Geometry check sheet. Reference: the model listing, model coordinates, mm. Face numbers are marked on the shaded views. A direction names the side the tool comes from. Round coordinates to 2 decimals unless told otherwise and drop trailing zeros. Order: outer loops, then holes, each group sorted by start corner. A loop starts at its lowest first (then second) coordinate and runs counter-clockwise, first axis right, second up. Notation, with made-up numbers: (28, 7) - (53, 7) arc R12 cw to (53, 19) - close; hole circle Ø11 at (59.25, 44). An arc over 180 degrees is marked (long way). Return JSON: item names as keys, results as strings. Group by question number.
Q1. Sectioned sample at B-B, the plane y = 42. Record the cut outline in (x, z).
Q2. Sectioned sample at C-C, the plane z = 4. Record the cut outline in (x, y).
Q3. Sectioned sample at D-D, the plane x = -6.5. Record the cut outline in (y, z).
Q4. Material ranges on line 1 along Y through (x, z) = (-4.25, -5); line 2 along Z through (x, y) = (-6.25, 16.5); line 3 along X through (y, z) = (48, 1.75), recorded low to high.
Q5. Gauge pin test, flat ends, axial feed: pin 1 Ø4 at (y, z) = (21.5, 4) entering from -X; pin 2 Ø3 at (y, z) = (28.5, 2.5) entering from +X (3 decimals); pin 3 Ø2 at (y, z) = (28.5, -3) entering from +X. Record the tip position at first contact, or that the pin passes through.
Q6. Tool access check on the marked faces 1, 2 and 3. Record the directions out of +Z, -Z, +X, -X, +Y, -Y that give a thin tool (end or side, any length) a straight path to the whole face; none if there is none.
Q7. Sectioned sample at A-A, the plane x = 0. Record the cut outline in (y, z), then the cut area to 3 significant figures.
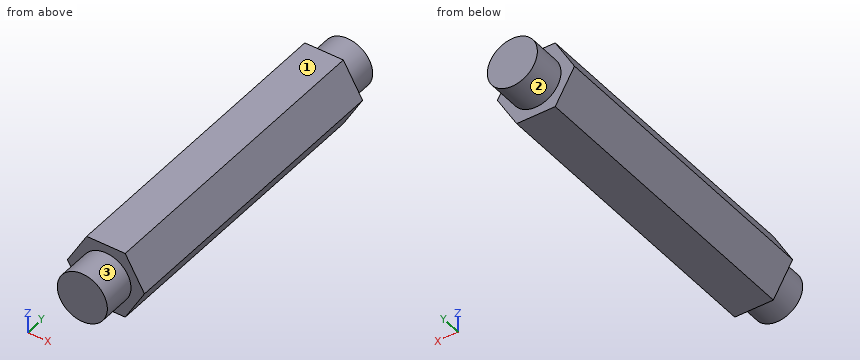
```python
from build123d import *

# Parameters (mm, degrees)
SALIENTE_EXTRUIR1_DEPTH = 58.68
CROQUIS2_R              = 4.7625
SALIENTE_EXTRUIR2_DEPTH = 6.35
SALIENTE_EXTRUIR3_START = 6.35
CROQUIS3_R              = 4.7625
SALIENTE_EXTRUIR3_DEPTH = 6.35


with BuildPart() as part:
    # Croquis1 → Saliente-Extruir1 (new body)
    with BuildSketch(Plane(origin=(0, 0, 0), x_dir=(1, 0, 0), z_dir=(0, 1, 0))):
        Polygon((7.332348419, 0), (3.666174209, 6.35), (-3.666174209, 6.35), (-7.332348419, 0), (-3.666174209, -6.35), (3.666174209, -6.35), align=None)
    extrude(amount=SALIENTE_EXTRUIR1_DEPTH)

    # Croquis2 → Saliente-Extruir2 (add)
    with BuildSketch(Plane(origin=(0, 58.68, 0), x_dir=(1, 0, 0), z_dir=(0, 1, 0))):
        with Locations(Location((0, 0, 0), (0, 0, 270))):
            Circle(CROQUIS2_R)
    extrude(amount=SALIENTE_EXTRUIR2_DEPTH)

    # Croquis3 → Saliente-Extruir3 (add)
    with BuildSketch(Plane.XZ.offset(SALIENTE_EXTRUIR3_START)):
        with Locations(Location((0, 0, 0), (0, 0, 90))):
            Circle(CROQUIS3_R)
    extrude(amount=-SALIENTE_EXTRUIR3_DEPTH)


solid = part.part
```
Reply:
{
 "1": {"outline": "(-7.33, 0) - (-3.67, -6.35) - (3.67, -6.35) - (7.33, 0) - (3.67, 6.35) - (-3.67, 6.35) - close"},
 "2": {"outline": "(-5.02, 0) - (-2.58, 0) - (-2.58, -6.35) - (2.58, -6.35) - (2.58, 0) - (5.02, 0) - (5.02, 58.68) - (2.58, 58.68) - (2.58, 65.03) - (-2.58, 65.03) - (-2.58, 58.68) - (-5.02, 58.68) - close"},
 "3": {"outline": "(0, -1.44) - (58.68, -1.44) - (58.68, 1.44) - (0, 1.44) - close"},
 "4": {"line 1": "0 to 58.68", "line 2": "-1.87 to 1.87", "line 3": "-6.32 to 6.32"},
 "5": {"pin 1": "x = -6.18", "pin 2": "x = 6.755", "pin 3": "x = 6.18"},
 "6": {"face 1": "+Z, +X, -X, +Y, -Y", "face 2": "+Y", "face 3": "-Y"},
 "7": {"outline": "(-6.35, -4.76) - (0, -4.76) - (0, -6.35) - (58.68, -6.35) - (58.68, -4.76) - (65.03, -4.76) - (65.03, 4.76) - (58.68, 4.76) - (58.68, 6.35) - (0, 6.35) - (0, 4.76) - (-6.35, 4.76) - close", "area": "866 mm^2"}
}
